Autodesk Inventor part; units mm, degrees
ref_plane "YZ Plane" through (0, 0, 0) normal (1, 0, 0) x (0, 1, 0)
ref_plane "XZ Plane" through (0, 0, 0) normal (0, 1, 0) x (-1, 0, 0)
ref_plane "XY Plane" through (0, 0, 0) normal (0, 0, 1) x (1, 0, 0)
sketch "Sketch1" plane through (0, 0, 0) normal (0, 0, 1) x (1, 0, 0)
  circle A0 centre (0, 0) radius 3
  dimension "d0" = 6
extrude "Extrusion1" add sketch "Sketch1" along normal blind 10
sketch "Sketch2" plane through (0, 0, 10) normal (0, 0, 1) x (1, 0, 0)
  circle A0 centre (0, 0) radius 3
  line L0 (1.3157, 2.1001) -> (2.4766, -0.0894)
  line L1 (2.4766, -0.0894) -> (1.1609, -2.1895)
  line L2 (1.1609, -2.1895) -> (-1.3157, -2.1001)
  line L3 (-1.3157, -2.1001) -> (-2.4766, 0.0894)
  line L4 (-2.4766, 0.0894) -> (-1.1609, 2.1895)
  line L5 (-1.1609, 2.1895) -> (1.3157, 2.1001)
extrude "Extrusion2" cut sketch "Sketch2" against normal blind 3 contours L0 L1 L2 L3 L4 L5
fillet "Fillet1" radius 0.3 1 edges at (-3, 0, 10)
properties part number "4"
Can you work these out from the model? Positions are in its coordinate system, mm. Round coordinates to 2 decimals unless told otherwise and drop trailing zeros. Loops run counter-clockwise (first coordinate to the right, second up) from the corner with the lowest first, then second, coordinate; pieces in that order, holes last. Notation, with made-up numbers: (8.25, 37.25) - (64.25, 37.25) arc R32 cw to (64.25, 63.25) - close; hole circle Ø5 at (57.25, -10). An arc over 180 degrees is marked (long way). Answer in a Markdown table with one row per item. Add a question column.
Q1. I want a section at A-A on z = 1.25. List the corners of the cut face in (x, y) for me, and give its area (3 significant figures).
Q2. I need wall thicknesses on L1, parallel to Z at x = 1, y = -0.25; L2, parallel to Y at x = -1, z = 8.5; L3, parallel to Y at x = 1.25, z = 8.25. Which ranges of each line are inside material? Lowest first, please.
Q3. We'd pull the mould along X, two halves only. Please class faces 1 (the flat face through (0, 0, 0)), 2 (the flat face through (0.06, 2.145, 8.521)), 3 (the cylindrical face through (-3, 0, 5)): pulls with the +X half, pulls with the -X half, needs draft (parallel to the pull), parting line crosses it, or undercut.
Q4. I want a section at B-B on x = 0. List the corners of the cut face in (y, z) for me.
Q5. For pin 1 Ø1 at (y, z) = (1, 8) entering from -X, with a flat end and sliding along its axis, tell me the tip position at first contact or that it passes through.
A:
| question | item | result |
|---|---|---|
| 1 | outline | circle Ø6 at (0, 0) |
| 1 | area | 28.3 mm^2 |
| 2 | L1 | 0 to 7 |
| 2 | L2 | -2.83 to -2.11, 2.18 to 2.83 |
| 2 | L3 | -2.73 to -2.05, 2.1 to 2.73 |
| 3 | face 1 | needs draft |
| 3 | face 2 | undercut |
| 3 | face 3 | parting line crosses it |
| 4 | outline | (-3, 0) - (3, 0) - (3, 9.7) arc R0.3 ccw to (2.7, 10) - (2.15, 10) - (2.15, 7) - (-2.15, 7) - (-2.15, 10) - (-2.7, 10) arc R0.3 ccw to (-3, 9.7) - close |
| 5 | pin 1 | x = -2.96 |
